CAD build for the part. Positions are in the model's coordinates, mm. A direction names the side the tool comes from. Give positions to 0.01 mm unless a question says otherwise; leave off trailing zeros. Order: outer loops, then holes, each group sorted by start corner. A loop starts at its lowest first (then second) coordinate and runs counter-clockwise, first axis right, second up.
Item 1: Band-saw the part on A-A on z = 31. Give the cut face in (x, y).
Item 2: Band-saw the part on B-B on z = -47. Give the cut face in (x, y).
Item 3: Flat gauge pins, fed straight in: P1, Ø22, axis at x = 2, z = 4, coming from the +Y side; P2, Ø18.5, axis at x = 80, y = 0, coming from the +Z side; P3, Ø12, axis at x = 92, z = -30, coming from the +Y side. Where does each tip first touch, or does it go through?
Item 4: Which spindle directions (+Z, -Z, +X, -X, +Y, -Y) get a long thin tool onto all of the face, cutting with end or side? Do faces 4 (the flat face through (-35.5, 42.57, 50.07)), 5 (the flat face through (90, -15, -27)), 6 (the cylindrical face through (-20, -15, 1)). Say none if no direction does.
Item 5: Band-saw the part on D-D on x = 48.5. Give the cut face in (y, z), plus the area to 3 significant figures.
Item 6: Band-saw the part on C-C on z = 0. Give the cut face in (x, y).
Item 7: Two-plate mould, pull along Z, no slides. Class faces 1 (the flat face through (-42.28, 35.21, -50.07)), 2 (the flat face through (-33, 25, 55)), 3 (the cylindrical face through (50.7, 0.66, 14.985)): released by +Z, released by -Z, zero draft, split by the parting line, or undercut.
Item 8: Wall check: L1, parallel to Z at x = 21, y = 1; L2, parallel to Y at x = 41, z = 0; L3, parallel to X at y = 4, z = 31. Give the ranges that are in metal, low to high.
```python
from build123d import *

# Parameters (mm, degrees)
SKETCH1_R               = 25
BOSS_EXTRUDE1_DEPTH     = 75
BOSS_EXTRUDE2_START     = 35
SKETCH3_R               = 10
BOSS_EXTRUDE2_DEPTH     = 35
BOSS_EXTRUDE2_DRAFT     = 16
SKETCH4_R               = 25
BOSS_EXTRUDE3_DEPTH     = 100
BOSS_EXTRUDE4_DEPTH     = 35
BOSS_EXTRUDE5_START     = 10
BOSS_EXTRUDE5_DEPTH     = 10
CUT_EXTRUDE2_DEPTH      = 190.22462748
CUT_EXTRUDE2_DEPTH_BACK = 190.22462748
SKETCH2_R               = 15
SKETCH7_R               = 15
CUT_EXTRUDE3_DEPTH      = 100
CUT_EXTRUDE4_DEPTH      = 160.392470452
CUT_EXTRUDE4_DEPTH_BACK = 160.392470452
SKETCH8_R               = 8
SKETCH9_R               = 5
CUT_EXTRUDE5_DEPTH      = 30


with BuildPart() as part:
    # Sketch1 → Boss-Extrude1 (new, symmetric)
    with BuildSketch(Plane.XY):
        Circle(SKETCH1_R)
    extrude(amount=BOSS_EXTRUDE1_DEPTH, both=True)


with BuildPart() as boss_extrude2_tool:
    # Sketch3 → Boss-Extrude2 (with draft: the straight prism first)
    with BuildSketch(Plane(origin=(0, 0, 0), x_dir=(1, 0, 0), z_dir=(0, 1, 0)).offset(BOSS_EXTRUDE2_START)):
        Circle(SKETCH3_R)
    extrude(amount=-BOSS_EXTRUDE2_DEPTH)
    # Boss-Extrude2: the draft: its side faces are tilted about the plane it starts from
    boss_extrude2_sides = [boss_extrude2_tool.faces().sort_by_distance(p)[0] for p in [
        (-10, 17.5, 0),
    ]]
    draft(boss_extrude2_sides, Plane(origin=(0, 0, 0), x_dir=(1, 0, 0), z_dir=(0, 1, 0)).offset(BOSS_EXTRUDE2_START), BOSS_EXTRUDE2_DRAFT)


with BuildPart() as part_1:
    add(part.part)

    # Boss-Extrude2: add boss_extrude2_tool
    add(boss_extrude2_tool.part)

    # Sketch4 → Boss-Extrude3 (add)
    with BuildSketch(Plane(origin=(0, 0, 0), x_dir=(0, 0, -1), z_dir=(1, 0, 0))):
        Circle(SKETCH4_R)
    extrude(amount=BOSS_EXTRUDE3_DEPTH)

    # Sketch5 → Boss-Extrude4 (add, symmetric)
    with BuildSketch(Plane.XY):
        with BuildLine():
            Line((80, 15), (100, 15))
            Line((100, 15), (100, -15))
            Line((100, -15), (80, -15))
            ThreePointArc((80, -15), (65, 0), (80, 15))
        make_face()
    extrude(amount=BOSS_EXTRUDE4_DEPTH, both=True)

    # Sketch6 → Boss-Extrude5 (add)
    with BuildSketch(Plane.XY.offset(45).offset(BOSS_EXTRUDE5_START)):
        with BuildLine():
            ThreePointArc((-45.383782434, 56.358781853), (-55.154328933, 55.154328933), (-56.358781853, 45.383782434))
            Line((-56.358781853, 45.383782434), (-21.441584906, -12.855288278))
            ThreePointArc((-21.441584906, -12.855288278), (-24.812182391, 3.058693344), (-17.67766953, 17.67766953))
            ThreePointArc((-17.67766953, 17.67766953), (-3.058693344, 24.812182391), (12.855288278, 21.441584906))
            Line((12.855288278, 21.441584906), (-45.383782434, 56.358781853))
        make_face()
        with BuildLine():
            ThreePointArc((-24.748737342, 31.819805153), (-23.284271247, 28.284271247), (-24.748737342, 24.748737342))
            ThreePointArc((-24.748737342, 24.748737342), (-28.284271247, 23.284271247), (-31.819805153, 24.748737342))
            Line((-31.819805153, 24.748737342), (-53.033008589, 45.961940777))
            ThreePointArc((-53.033008589, 45.961940777), (-53.033008589, 53.033008589), (-45.961940777, 53.033008589))
            Line((-45.961940777, 53.033008589), (-24.748737342, 31.819805153))
        make_face(mode=Mode.SUBTRACT)
    boss_extrude5 = extrude(amount=-BOSS_EXTRUDE5_DEPTH)

    # Mirror1: Boss-Extrude5 across plane
    add(boss_extrude5.mirror(Plane.XY))

    # Sketch2 → Cut-Extrude2 (cut, two sides: drawn at the far end of the back side and taken through both)
    with BuildSketch(Plane.XY.offset(75).offset(-CUT_EXTRUDE2_DEPTH_BACK)):
        Circle(SKETCH2_R)
    extrude(amount=CUT_EXTRUDE2_DEPTH + CUT_EXTRUDE2_DEPTH_BACK, mode=Mode.SUBTRACT)

    # Sketch7 → Cut-Extrude3 (cut)
    with BuildSketch(Plane(origin=(100, 0, 0), x_dir=(0, 0, -1), z_dir=(1, 0, 0))):
        Circle(SKETCH7_R)
    extrude(amount=-CUT_EXTRUDE3_DEPTH, mode=Mode.SUBTRACT)

    # Sketch8 → Cut-Extrude4 (cut, two sides: drawn at the far end of the back side and taken through both)
    with BuildSketch(Plane.XY.offset(35).offset(-CUT_EXTRUDE4_DEPTH_BACK)):
        with Locations((80, 0)):
            Circle(SKETCH8_R)
    extrude(amount=CUT_EXTRUDE4_DEPTH + CUT_EXTRUDE4_DEPTH_BACK, mode=Mode.SUBTRACT)

    # Sketch9 → Cut-Extrude5 (cut)
    with BuildSketch(Plane(origin=(0, 35, 0), x_dir=(1, 0, 0), z_dir=(0, 1, 0))):
        with Locations(Location((0, 0, 0), (0, 0, 270))):
            Circle(SKETCH9_R)
    extrude(amount=-CUT_EXTRUDE5_DEPTH, mode=Mode.SUBTRACT)


solid = part_1.part
```
The answers:
1. outline: circle Ø50 at (0, 0); (80, -15) - (100, -15) - (100, 15) - (80, 15) arc R15 ccw to start; hole circle Ø30 at (0, 0); hole circle Ø16 at (80, 0)
2. outline: (-56.36, 45.38) - (-21.44, -12.86) arc R25 ccw (long way) to (12.86, 21.44) - (-45.38, 56.36) arc R8 ccw to start; hole (-53.03, 45.96) - (-31.82, 24.75) arc R5 ccw to (-24.75, 31.82) - (-45.96, 53.03) arc R5 ccw to start; hole circle Ø30 at (0, 0)
3. P1: stops at y = 35
3. P2: stops at z = 35
3. P3: stops at y = 15
4. face 4: +Z, -Z
4. face 5: -Z, +X, -Y
4. face 6: none
5. outline: circle Ø50 at (0, 0); hole circle Ø30 at (0, 0)
5. area: 1,260 mm2
6. outline: (-14.12, 20.63) arc R25 ccw to (0, -25) - (100, -25) - (100, -15) - (0, -15) arc R15 cw to (-5, 14.14) - (-5, 35) - (-10, 35) - close; (5, 15) - (100, 15) - (100, 25) - (12.87, 25) - (10, 35) - (5, 35) - close
7. face 1: zero draft
7. face 2: released by +Z
7. face 3: undercut
8. L1: z = -75 to -14.97, 14.97 to 75
8. L2: y = -25 to -15, 15 to 25
8. L3: x = -24.68 to -14.46, 14.46 to 24.68, 65.54 to 73.07, 86.93 to 100
